Here's how the part is built. I have some questions about the finished solid (model axes, mm). A direction names the side the tool comes from. Round coordinates to 2 decimals unless told otherwise and drop trailing zeros. Write each loop counter-clockwise with the first axis right and the second up, starting at its lowest first coordinate (ties: lowest second). Pieces come first, ordered by that corner, then holes. Notation, with made-up numbers: (-7, -35.75) -> (36, -35.75) arc R20 cw to (36, -3.75) -> close; hole circle Ø6 at (11.5, 53.25). An arc over 180 degrees is marked (long way). Answer in a Markdown table with one row per item.
from build123d import *

# Parameters (mm, degrees)
SKETCH_1_R          = 35
SKETCH_1_R_2        = 32.5
EXTRUDE_1_DEPTH     = 10
EXTRUDE_2_DEPTH     = 50
CUT_EXTRUDE_1_REACH = 118.001
SKETCH_3_R          = 4
CUT_EXTRUDE_2_REACH = 120.373
SKETCH_4_R          = 1.7
CUT_EXTRUDE_3_REACH = 120.373
SKETCH_5_R          = 1.7


with BuildPart() as part:
    # ｽｹｯﾁ1 → ﾎﾞｽ - 押し出し1 (new body)
    with BuildSketch(Plane.XY):
        Circle(SKETCH_1_R)
        Circle(SKETCH_1_R_2, mode=Mode.SUBTRACT)
    extrude(amount=EXTRUDE_1_DEPTH)

    # ｽｹｯﾁ2 → ﾎﾞｽ - 押し出し2 (add)
    with BuildSketch(Plane(origin=(0, 0, 0), x_dir=(-1, 0, 0), z_dir=(0, 0, -1))):
        Polygon((0, -32.5), (-70, -32.5), (-70, -36.5), (80, -36.5), (80, -32.5), align=None)
    extrude(amount=-EXTRUDE_2_DEPTH)

    # ｽｹｯﾁ3 → ｶｯﾄ - 押し出し1 (cut, up to next)
    with BuildSketch(Plane(origin=(0, -32.5, 0), x_dir=(1, 0, 0), z_dir=(0, 1, 0)), mode=Mode.PRIVATE) as cut_extrude_1_sk1:
        with Locations(Location((48, -25, 0), (0, 0, 180))):
            Circle(SKETCH_3_R)
    cut_extrude_1_tool1 = extrude(cut_extrude_1_sk1.sketch, amount=-CUT_EXTRUDE_1_REACH, mode=Mode.PRIVATE) & part.part
    add(cut_extrude_1_tool1.solids().sort_by_distance((48, -32.5, 25))[0], mode=Mode.SUBTRACT)

    # ｽｹｯﾁ4 → ｶｯﾄ - 押し出し2 (cut, up to next)
    with BuildSketch(Plane.XZ.offset(36.5), mode=Mode.PRIVATE) as cut_extrude_2_sk1:
        with Locations(Location((63.5, 40.5, 0), (0, 0, 270))):
            Circle(SKETCH_4_R)
    cut_extrude_2_tool1 = extrude(cut_extrude_2_sk1.sketch, amount=-CUT_EXTRUDE_2_REACH, mode=Mode.PRIVATE) & part.part
    # ｽｹｯﾁ4 → ｶｯﾄ - 押し出し2 (cut, up to next)
    with BuildSketch(Plane.XZ.offset(36.5), mode=Mode.PRIVATE) as cut_extrude_2_sk2:
        with Locations(Location((63.5, 9.5, 0), (0, 0, 270))):
            Circle(SKETCH_4_R)
    cut_extrude_2_tool2 = extrude(cut_extrude_2_sk2.sketch, amount=-CUT_EXTRUDE_2_REACH, mode=Mode.PRIVATE) & part.part
    # ｽｹｯﾁ4 → ｶｯﾄ - 押し出し2 (cut, up to next)
    with BuildSketch(Plane.XZ.offset(36.5), mode=Mode.PRIVATE) as cut_extrude_2_sk3:
        with Locations(Location((32.5, 40.5, 0), (0, 0, 270))):
            Circle(SKETCH_4_R)
    cut_extrude_2_tool3 = extrude(cut_extrude_2_sk3.sketch, amount=-CUT_EXTRUDE_2_REACH, mode=Mode.PRIVATE) & part.part
    # ｽｹｯﾁ4 → ｶｯﾄ - 押し出し2 (cut, up to next)
    with BuildSketch(Plane.XZ.offset(36.5), mode=Mode.PRIVATE) as cut_extrude_2_sk4:
        with Locations(Location((32.5, 9.5, 0), (0, 0, 270))):
            Circle(SKETCH_4_R)
    cut_extrude_2_tool4 = extrude(cut_extrude_2_sk4.sketch, amount=-CUT_EXTRUDE_2_REACH, mode=Mode.PRIVATE) & part.part
    add(cut_extrude_2_tool1.solids().sort_by_distance((63.5, -36.5, 40.5))[0], mode=Mode.SUBTRACT)
    add(cut_extrude_2_tool2.solids().sort_by_distance((63.5, -36.5, 9.5))[0], mode=Mode.SUBTRACT)
    add(cut_extrude_2_tool3.solids().sort_by_distance((32.5, -36.5, 40.5))[0], mode=Mode.SUBTRACT)
    add(cut_extrude_2_tool4.solids().sort_by_distance((32.5, -36.5, 9.5))[0], mode=Mode.SUBTRACT)

    # ｽｹｯﾁ5 → ｶｯﾄ - 押し出し3 (cut, up to next)
    with BuildSketch(Plane.XZ.offset(36.5), mode=Mode.PRIVATE) as cut_extrude_3_sk1:
        with Locations(Location((-75, 42.5, 0), (0, 0, 270))):
            Circle(SKETCH_5_R)
    cut_extrude_3_tool1 = extrude(cut_extrude_3_sk1.sketch, amount=-CUT_EXTRUDE_3_REACH, mode=Mode.PRIVATE) & part.part
    # ｽｹｯﾁ5 → ｶｯﾄ - 押し出し3 (cut, up to next)
    with BuildSketch(Plane.XZ.offset(36.5), mode=Mode.PRIVATE) as cut_extrude_3_sk2:
        with Locations(Location((-75, 7.5, 0), (0, 0, 270))):
            Circle(SKETCH_5_R)
    cut_extrude_3_tool2 = extrude(cut_extrude_3_sk2.sketch, amount=-CUT_EXTRUDE_3_REACH, mode=Mode.PRIVATE) & part.part
    add(cut_extrude_3_tool1.solids().sort_by_distance((-75, -36.5, 42.5))[0], mode=Mode.SUBTRACT)
    add(cut_extrude_3_tool2.solids().sort_by_distance((-75, -36.5, 7.5))[0], mode=Mode.SUBTRACT)


solid = part.part
1) I want a section at B-B, the plane z = 25. List the corners of the cut face in (x, y) for me, and give its area (3 significant figures).
Response:
| item | result |
|---|---|
| outline | (-80, -36.5) -> (44, -36.5) -> (44, -32.5) -> (-80, -32.5) -> close; (52, -36.5) -> (70, -36.5) -> (70, -32.5) -> (52, -32.5) -> close |
| area | 568 mm^2 |
2) I need wall thicknesses on line 1 (X direction, y = -35.6, z = 40.5); line 2 (X direction, y = -34.3, z = 7.5); line 3 (X direction, y = -35, z = 9). Which ranges of each line are inside material? Lowest first, please. Write a range as [from, to].
Response:
| item | result |
|---|---|
| line 1 | x = [-80, 30.8], [34.2, 61.8], [65.2, 70] |
| line 2 | x = [-80, -76.7], [-73.3, 70] |
| line 3 | x = [-80, -75.8], [-74.2, 30.88], [34.12, 61.88], [65.12, 70] |
3) For pin 1 (5.5 mm diameter, centred on x = 63.5, z = 9.5, fed in from +Y), with a flat end and sliding along its axis, tell me the tip position at first contact or that it passes through.
Response:
| item | result |
|---|---|
| pin 1 | stops at y = -32.5 |
4) Which directions (+Z, -Z, +X, -X, +Y, -Y) give clear straight access to the entire face, cutting with the end or side of a thin tool? Please do faces 4 (the face through (15.4, 28.9, 10)), 5 (the face through (30.84, -34.53, 9.87)), 6 (the face through (-4.6, -32.4, 0)).
Response:
| item | result |
|---|---|
| face 4 | +Z, +X, -X, +Y |
| face 5 | -Y |
| face 6 | -Z, +X, -X, +Y, -Y |
5) We'd pull the mould along Y, two halves only. Please class faces 1 (the face through (1.353, 34.974, 4.93)), 2 (the face through (64.65, -34.53, 41.75)), 3 (the face through (-4, -36.5, 25)): +Y half, -Y half, draft (parallel to the pull), parting line (faces both ways), or undercut.
Response:
| item | result |
|---|---|
| face 1 | undercut |
| face 2 | draft |
| face 3 | -Y half |
6) I want a section at C-C, the plane y = 0. List the corners of the cut face in (x, z) for me, and give its area (3 significant figures).
Response:
| item | result |
|---|---|
| outline | (-35, 0) -> (-32.5, 0) -> (-32.5, 10) -> (-35, 10) -> close; (32.5, 0) -> (35, 0) -> (35, 10) -> (32.5, 10) -> close |
| area | 50.0 mm^2 |
7) I want a section at D-D, the plane x = 3. List the corners of the cut face in (y, z) for me, and give its area (3 significant figures).
Response:
| item | result |
|---|---|
| outline | (-36.5, 0) -> (-32.36, 0) -> (-32.36, 10) -> (-32.5, 10) -> (-32.5, 50) -> (-36.5, 50) -> close; (32.36, 0) -> (34.87, 0) -> (34.87, 10) -> (32.36, 10) -> close |
| area | 226 mm^2 |
8) I want a section at A-A, the plane x = 63.5. List the corners of the cut face in (y, z) for me, and give its area (3 significant figures).
Response:
| item | result |
|---|---|
| outline | (-36.5, 0) -> (-32.5, 0) -> (-32.5, 7.8) -> (-36.5, 7.8) -> close; (-36.5, 11.2) -> (-32.5, 11.2) -> (-32.5, 38.8) -> (-36.5, 38.8) -> close; (-36.5, 42.2) -> (-32.5, 42.2) -> (-32.5, 50) -> (-36.5, 50) -> close |
| area | 173 mm^2 |
